Part model, mm, in its own coordinate system. Coordinates: 2 decimals unless noted, no trailing zeros. Write each loop counter-clockwise with the first axis right and the second up, starting at its lowest first coordinate (ties: lowest second). Pieces come first, ordered by that corner, then holes. Notation, with made-up numbers: (-28, 20) - (4, 20) arc R25 ccw to (4, 57) - close; hole circle Ø3 at (61.25, 64.5). An arc over 180 degrees is marked (long way). Use a Markdown table: item, result.
```python
from build123d import *

# Parameters (mm, degrees)
SKETCH_1_W          = 7.7
SKETCH_1_H          = 5.3
EXTRUDE_1_DEPTH     = 1
CUT_EXTRUDE_1_DEPTH = 1


with BuildPart() as part:
    # 草图1 → 凸台-拉伸1 (new body)
    with BuildSketch(Plane(origin=(0, 0, 0), x_dir=(0, 0, -1), z_dir=(1, 0, 0))):
        Rectangle(SKETCH_1_W, SKETCH_1_H)
    extrude(amount=EXTRUDE_1_DEPTH)

    # 草图2 → 切除-拉伸1 (cut)
    with BuildSketch(Plane(origin=(1, 0, 0), x_dir=(0, 0, -1), z_dir=(1, 0, 0))):
        with BuildLine():
            Line((-3.85, -0.5), (-3.85, 0.5))
            ThreePointArc((-3.85, 0.5), (-3.35, 0), (-3.85, -0.5))
        make_face()
        with BuildLine():
            Line((3.85, -0.5), (3.85, 0.5))
            ThreePointArc((3.85, 0.5), (3.35, 0), (3.85, -0.5))
        make_face()
    extrude(amount=-CUT_EXTRUDE_1_DEPTH, mode=Mode.SUBTRACT)


solid = part.part
```
Item 1: Band-saw the part on B-B, the plane x = 0.1. Give the cut face in (y, z), then the cut area to 3 significant figures.
From the geometry:
| item | result |
|---|---|
| outline | (-2.65, -3.85) - (-0.5, -3.85) arc R0.5 cw to (0.5, -3.85) - (2.65, -3.85) - (2.65, 3.85) - (0.5, 3.85) arc R0.5 cw to (-0.5, 3.85) - (-2.65, 3.85) - close |
| area | 40.0 mm^2 |
Item 2: Band-saw the part on C-C, the plane y = 0. Give the cut face in (x, z).
From the geometry:
| item | result |
|---|---|
| outline | (0, -3.35) - (1, -3.35) - (1, 3.35) - (0, 3.35) - close |
Item 3: Band-saw the part on A-A, the plane z = 3.5. Give the cut face in (x, y), then the cut area to 3 significant figures.
From the geometry:
| item | result |
|---|---|
| outline | (0, -2.65) - (1, -2.65) - (1, -0.36) - (0, -0.36) - close; (0, 0.36) - (1, 0.36) - (1, 2.65) - (0, 2.65) - close |
| area | 4.59 mm^2 |
Item 4: Drill centre lines: probe 1 along Z at (x, y) = (0.7, 0); probe 2 along Y at (x, z) = (0.15, 3.5); probe 3 along Z at (x, y) = (0.65, -0.4). Where is each one in solid material? Low to high.
From the geometry:
| item | result |
|---|---|
| probe 1 | -3.35 to 3.35 |
| probe 2 | -2.65 to -0.36, 0.36 to 2.65 |
| probe 3 | -3.55 to 3.55 |
